The drawing under review shows one solid part. Ordinate dimensions are in mm from its lowest x, y, z. A direction names the side the tool comes from. Coordinates: 2 decimals unless noted, no trailing zeros. Write each loop counter-clockwise with the first axis right and the second up, starting at its lowest first coordinate (ties: lowest second). Pieces come first, ordered by that corner, then holes. Notation, with made-up numbers: (-13, -23.75) - (32, -23.75) arc R23 cw to (32, 1.25) - close; hole circle Ø4 at (4.5, 40.5). An arc over 180 degrees is marked (long way). Use a Markdown table: item, result.
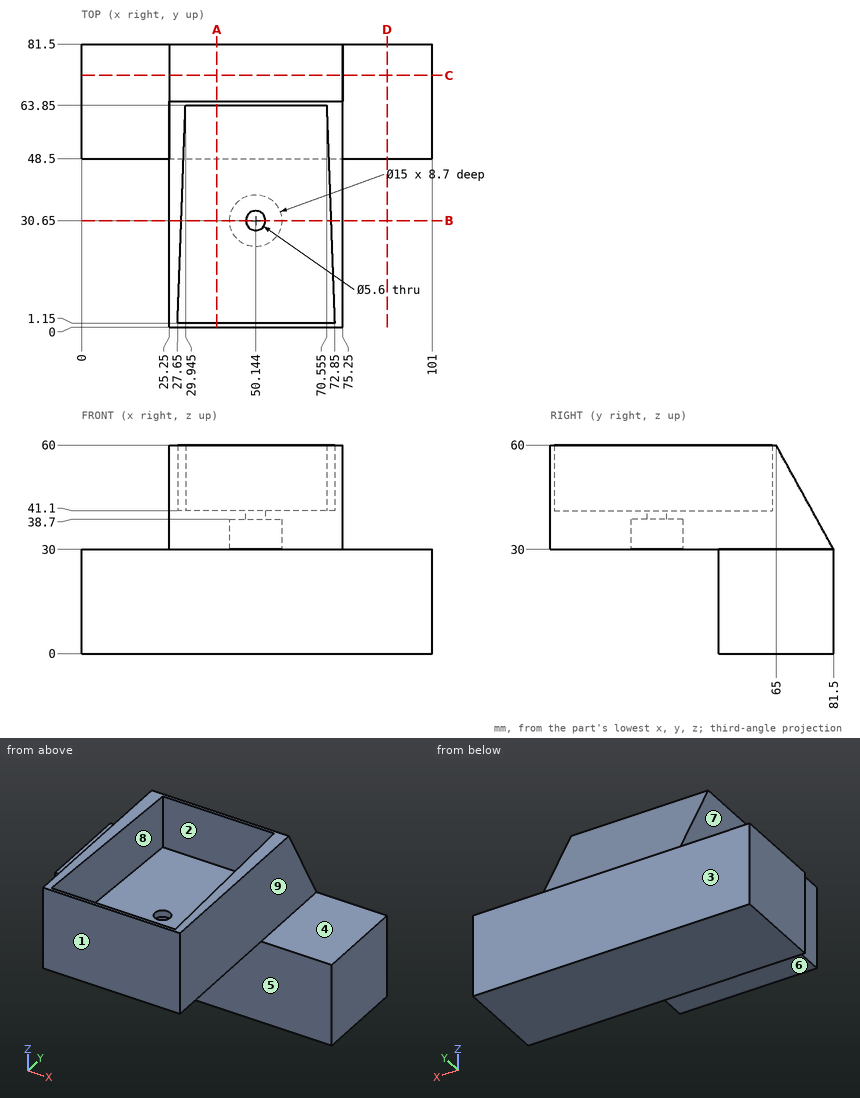
(1) Take a section at A-A on x = 39. Write out the cut boundary in (y, z).
Determined:
| item | result |
|---|---|
| outline | (0, 30) - (48.5, 30) - (48.5, 0) - (81.5, 0) - (81.5, 30) - (65, 60) - (63.85, 60) - (63.85, 41.1) - (1.15, 41.1) - (1.15, 60) - (0, 60) - close |
(2) Machinability: for the marked faces 1, 2, 3, 4 and 5, which of the approach directions +Z, -Z, +X, -X, +Y, -Y give a long, thin tool a straight path to every point of the face, cutting with its end or side? Answer none if there is none.
Determined:
| item | result |
|---|---|
| face 1 | +Z, -Z, +X, -X, -Y |
| face 2 | +Z |
| face 3 | +Z, -Z, +X, -X, +Y |
| face 4 | +Z, +X, +Y, -Y |
| face 5 | -Z, +X, -X, -Y |
(3) Take a section at D-D on x = 88. Write out the cut boundary in (y, z).
Determined:
| item | result |
|---|---|
| outline | (48.5, 0) - (81.5, 0) - (81.5, 30) - (48.5, 30) - close |
(4) For L1, parallel to X at y = 30, z = 35; L2, parallel to Z at x = 95.5, y = 76; L3, parallel to Y at x = 87, z = 19.5, list the stretches that pass through material, from the lowest coordinate up. Write a range as from..to.
Determined:
| item | result |
|---|---|
| L1 | 25.25..42.67, 57.62..75.25 |
| L2 | 0..30 |
| L3 | 48.5..81.5 |
(5) Take a section at B-B on y = 30.65. Write out the cut boundary in (x, z), and give its area (3 significant figures).
Determined:
| item | result |
|---|---|
| outline | (25.25, 30) - (42.64, 30) - (42.64, 38.7) - (47.34, 38.7) - (47.34, 41.1) - (28.73, 41.1) - (28.73, 60) - (25.25, 60) - close; (52.94, 38.7) - (57.64, 38.7) - (57.64, 30) - (75.25, 30) - (75.25, 60) - (71.77, 60) - (71.77, 41.1) - (52.94, 41.1) - close |
| area | 543 mm2 |
(6) Draft analysis for pull direction X (two halves, no side actions). For the marked faces 6, 7, 8 and 9, state which applies: +X half, -X half, draft (parallel to the pull), parting line (faces both ways), or undercut.
Determined:
| item | result |
|---|---|
| face 6 | draft |
| face 7 | -X half |
| face 8 | undercut |
| face 9 | +X half |
(7) For pin 1 (12 mm diameter, centred on x = 49, y = 30.5, fed in from -Z); pin 2 (3 mm diameter, centred on y = 45.5, z = 15.5, fed in from +X); pin 3 (12 mm diameter, centred on y = 65.5, z = 47, fed in from -X); pin 4 (17 mm diameter, centred on x = 50.14, y = 30.65, fed in from +Z), all flat-tipped, find the tip position at first contact; note any pin that passes through.
Determined:
| item | result |
|---|---|
| pin 1 | z = 38.7 |
| pin 2 | through |
| pin 3 | x = 25.25 |
| pin 4 | z = 41.1 |
(8) Take a section at C-C on y = 72.5. Write out the cut boundary in (x, z), and give its area (3 significant figures).
Determined:
| item | result |
|---|---|
| outline | (0, 0) - (101, 0) - (101, 30) - (75.25, 30) - (75.25, 46.36) - (25.25, 46.36) - (25.25, 30) - (0, 30) - close |
| area | 3,850 mm2 |
